Model file for the job. Use its own axes, mm. Face numbers are marked on the shaded views. A direction names the side the tool comes from. Give positions to 0.01 mm unless a question says otherwise; leave off trailing zeros. Loops run counter-clockwise (first coordinate to the right, second up) from the corner with the lowest first, then second, coordinate; pieces in that order, holes last. Notation, with made-up numbers: M 24,-11.5 L 43,-11.5 A12 ccw 43,-2.5 Z; hole C 3,62 d3. An arc over 180 degrees is marked long. Use CSV: the item, a comma, the result in double quotes. Start each with the question number.
(1) Slice it at A-A on x = 0. List the corners of the cut face in (y, z) (3 decimals), and give its area (3 significant figures).
(2) Flat gauge pins, fed straight in: P1, Ø6, axis at x = 1, z = 0.5, coming from the -Y side; P2, Ø4, axis at x = -3, y = 7.5, coming from the +Z side; P3, Ø2, axis at x = 0, z = -0.5, coming from the -Y side; P4, Ø6, axis at x = 3, z = -1.5, coming from the +Y side. Where does each tip first touch, or does it go through?
(3) Tool access for the marked faces 1, 2 and 3: list every direction of +Z, -Z, +X, -X, +Y, -Y with a clear straight run to the whole face (end or side of a thin tool).
(4) Slice it at C-C on y = 2.75. List the corners of the cut face in (x, z).
(5) Slice it at B-B on z = 0. List the corners of the cut face in (x, y), and give its area (3 significant figures).
(6) Wall check: line 1 along X through (y, z) = (3.15, 0); line 2 along X through (y, z) = (1.25, -3.25); line 3 along Z through (x, y) = (-3.25, 6). Give the ranges that are in metal, low to high. Write a range as from..to.
(7) Two-plate mould, pull along X, no slides. Class the marked faces 4, 5 and 6: pulls with the +X half, pulls with the -X half, needs draft (parallel to the pull), parting line crosses it, or undercut.
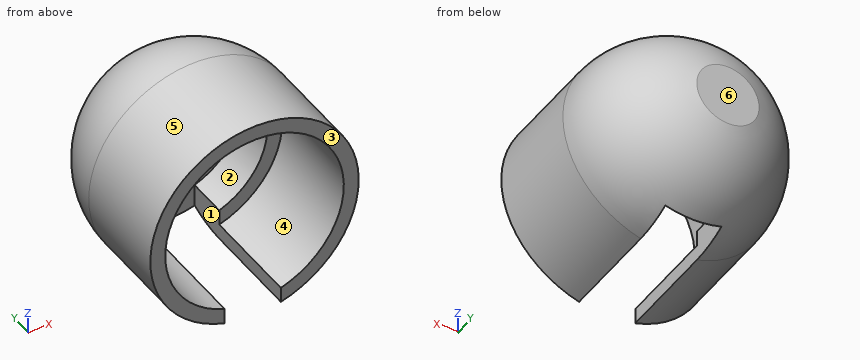
```python
from build123d import *

# Parameters (mm, degrees)
SKETCH1_R           = 5.25
SKETCH1_R_2         = 4.5
BOSS_EXTRUDE1_DEPTH = 5
CUT_EXTRUDE1_DEPTH  = 5
CUT_EXTRUDE2_DEPTH  = 2
SKETCH6_R           = 2
CUT_EXTRUDE4_DEPTH  = 0.35


with BuildPart() as part:
    # Sketch1 → Boss-Extrude1 (new body)
    with BuildSketch(Plane(origin=(0, 0, 0), x_dir=(1, 0, 0), z_dir=(0, 1, 0))):
        Circle(SKETCH1_R)
        Circle(SKETCH1_R_2, mode=Mode.SUBTRACT)
    extrude(amount=BOSS_EXTRUDE1_DEPTH)

    # Sketch2 → Cut-Extrude1 (cut)
    with BuildSketch(Plane(origin=(0, 0, 0), x_dir=(1, 0, 0), z_dir=(0, 1, 0))):
        Polygon((1.327689147, 3.795637322), (1.327689147, 5.701107087), (-1.5, 5.701107087), (-1.5, 3.701107087), align=None)
    extrude(amount=CUT_EXTRUDE1_DEPTH, mode=Mode.SUBTRACT)

    # Sketch4 → Revolve1 (revolve)
    with BuildSketch(Plane.XY):
        with BuildLine():
            Line((5.25, 5), (0, 5))
            Line((0, 5), (0, 10.18))
            ThreePointArc((0, 10.18), (3.687644912, 8.667004979), (5.25, 5))
        make_face()
    revolve(axis=Axis((0, 5, 0), (0, 1, 0)))

    # Sketch5 → Cut-Extrude2 (cut)
    with BuildSketch(Plane(origin=(0, 5, 0), x_dir=(-1, 0, 0), z_dir=(0, -1, 0))):
        with BuildLine():
            Line((1.5, 3.436931771), (1.5, 6))
            Line((1.5, 6), (-1.327689147, 6))
            Line((-1.327689147, 6), (-1.327689147, 3.507098734))
            ThreePointArc((-1.327689147, 3.507098734), (-0.093024772, -3.748846008), (1.5, 3.436931771))
        make_face()
    extrude(amount=-CUT_EXTRUDE2_DEPTH, mode=Mode.SUBTRACT)

    # Sketch6 → Cut-Extrude4 (cut)
    with BuildSketch(Plane(origin=(0, 10.29, 0), x_dir=(-1, 0, 0), z_dir=(0, -1, 0))):
        Circle(SKETCH6_R)
    extrude(amount=CUT_EXTRUDE4_DEPTH, mode=Mode.SUBTRACT)


solid = part.part
```
Reply:
1,outline,"M 0,4.5 L 5,4.5 L 5,3.75 L 7,3.75 L 7,-4.825 A5.25 ccw 9.94,-1.569 L 9.94,1.569 A5.25 ccw 5,5.25 L 0,5.25 Z"
1,area,"28.1 mm^2"
2,P1,"stops at y = 5"
2,P2,"stops at z = 4.87"
2,P3,"stops at y = 7"
2,P4,"stops at y = 9.94"
3,face 1,"-Z, -Y"
3,face 2,"-Y"
3,face 3,"+Z, -Z, +X, -X, -Y"
4,outline,"M -1.5,-5.03 L -1.5,-4.24 A4.5 cw long 1.33,-4.3 L 1.33,-5.08 A5.25 ccw long Z"
5,outline,"M -5.25,0 L -4.5,0 L -4.5,5 L -3.75,5 L -3.75,7 L 3.75,7 L 3.75,5 L 4.5,5 L 4.5,0 L 5.25,0 L 5.25,5 A5.25 ccw 1.57,9.94 L -1.57,9.94 A5.25 ccw -5.25,5 Z"
5,area,"34.6 mm^2"
6,line 1,"x = -5.25..-4.5, 4.5..5.25"
6,line 2,"x = -4.12..-3.11, 3.11..4.12"
6,line 3,"z = -3.98..-1.87, 1.87..3.98"
7,face 4,"undercut"
7,face 5,"parting line crosses it"
7,face 6,"needs draft"
